Part print with two shaded views. Sizes in mm from the minimum x, y, z corner. Round coordinates to 2 decimals unless told otherwise and drop trailing zeros. Write each loop counter-clockwise with the first axis right and the second up, starting at its lowest first coordinate (ties: lowest second). Pieces come first, ordered by that corner, then holes. Notation, with made-up numbers: (43.25, 17.5) -> (83.25, 17.5) arc R21 ccw to (83.25, 31.5) -> close; hole circle Ø7 at (68.5, 47). An arc over 180 degrees is marked (long way). Return JSON: item names as keys, results as strings. Group by question number.
(1) Saw through at B-B (y = 71). List the corners of the cut face in (x, z).
(2) Drop a flat-ended pin along its axis: pin 1 Ø3.5 at (x, y) = (95, 84) entering from +Z. Give the stop position or say it passes through.
(3) Drill centre lines: L1, parallel to X at y = 57.5, z = 1.2; L2, parallel to X at y = 29.5, z = 0.75; L3, parallel to Y at x = 74, z = 0.6. Where is each one in solid material? Low to high. Write a range as from..to.
(4) Saw through at C-C (z = 0.8). List the corners of the cut face in (x, y), plus the area to 3 significant figures.
(5) Saw through at A-A (y = 33). List the corners of the cut face in (x, z), plus the area to 3 significant figures.
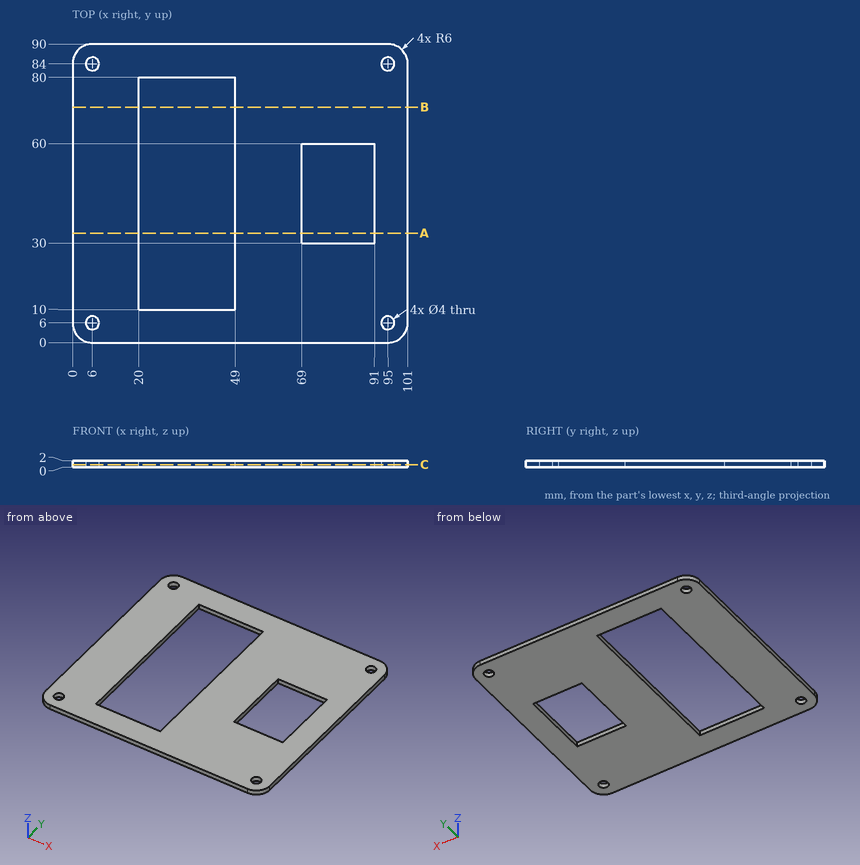
Computed values:
{
 "1": {"outline": "(0, 0) -> (20, 0) -> (20, 2) -> (0, 2) -> close; (49, 0) -> (101, 0) -> (101, 2) -> (49, 2) -> close"},
 "2": {"pin 1": "through"},
 "3": {"L1": "0..20, 49..69, 91..101", "L2": "0..20, 49..101", "L3": "0..30, 60..90"},
 "4": {"outline": "(0, 6) arc R6 ccw to (6, 0) -> (95, 0) arc R6 ccw to (101, 6) -> (101, 84) arc R6 ccw to (95, 90) -> (6, 90) arc R6 ccw to (0, 84) -> close; hole circle Ø4 at (6, 6); hole circle Ø4 at (6, 84); hole (20, 10) -> (49, 10) -> (49, 80) -> (20, 80) -> close; hole (69, 30) -> (91, 30) -> (91, 60) -> (69, 60) -> close; hole circle Ø4 at (95, 6); hole circle Ø4 at (95, 84)", "area": "6,320 mm2"},
 "5": {"outline": "(0, 0) -> (20, 0) -> (20, 2) -> (0, 2) -> close; (49, 0) -> (69, 0) -> (69, 2) -> (49, 2) -> close; (91, 0) -> (101, 0) -> (101, 2) -> (91, 2) -> close", "area": "100 mm2"}
}
